Build history of the part. All positions in model axes, mm. A direction names the side the tool comes from. Give positions to 0.01 mm unless a question says otherwise; leave off trailing zeros. Order: outer loops, then holes, each group sorted by start corner. A loop starts at its lowest first (then second) coordinate and runs counter-clockwise, first axis right, second up. Notation, with made-up numbers: (-21, 77.5) - (-4, 77.5) arc R20 ccw to (-4, 107.5) - close; hole circle Ø2 at (42.25, 31.25). An arc over 180 degrees is marked (long way). Use a Markdown table: item, result.
Autodesk Fusion 360 part; units mm, degrees
sketch "Sketch1" plane through (0, 0, 0) normal (0, 0, 1) x (1, 0, 0)
  line L0 (55.4833, 22.0753) -> (95.4833, 22.0753)
  line L1 (95.4833, 22.0753) -> (95.4833, 19.0753)
  line L2 (95.4833, 19.0753) -> (55.4833, 19.0753)
  line L3 (55.4833, 19.0753) -> (55.4833, 22.0753)
  line L4 (95.4833, 22.0753) -> (98.8643, 14.8248)
  line L5 (98.8643, 14.8248) -> (97.7152, 14.289)
  line L6 (97.7152, 14.289) -> (95.4833, 19.0753)
  line L7 (55.4833, 19.0753) -> (50.4119, 29.951)
  line L8 (50.4119, 29.951) -> (51.561, 30.4868)
  line L9 (55.4833, 22.0753) -> (51.561, 30.4868)
  dimension "d2" = 3
  dimension "d3" = 40
  dimension "d5" = 115
  dimension "d8" = 115
  dimension "d9" = 115
  dimension "d10" = 115
  dimension "d12" = 8
  dimension "d13" = 12
extrude "Extrude1" add sketch "Sketch1" along normal blind 12
sketch "Sketch2" plane through (86.8847, 40.515, 0) normal (0.9063, 0.4226, 0) x (-0.4226, 0.9063, 0)
  line L0 (-28.346, 0) -> (-20.346, 0)
  line L1 (-20.346, 0) -> (-20.346, 12)
  line L2 (-20.346, 12) -> (-28.346, 12)
  line L3 (-28.346, 12) -> (-28.346, 0)
  line L4 (-25.346, 12) -> (-25.346, 0) construction
  line L5 (-20.346, 6) -> (-28.346, 6) construction
  circle A0 centre (-25.346, 6) radius 1.1
  dimension "d17" = 2.2
  dimension "d23" = 3
extrude "Extrude2" cut sketch "Sketch2" against normal up to surface (1.2679 mm away) contours A0
sketch "Sketch4" plane through (54.029, 25.1941, 0) normal (0.9063, 0.4226, 0) x (-0.4226, 0.9063, 0)
  line L0 (-3.4413, 0) -> (5.8398, 0)
  line L1 (5.8398, 0) -> (5.8398, 12)
  line L2 (5.8398, 12) -> (-3.4413, 12)
  line L3 (-3.4413, 12) -> (-3.4413, 0)
  line L4 (1.1993, 12) -> (1.1993, 0) construction
  line L5 (5.8398, 6) -> (-3.4413, 6) construction
  circle A0 centre (1.1993, 6) radius 1
  dimension "d24" = 2
extrude "Extrude3" cut sketch "Sketch4" against normal up to surface (1.2679 mm away) contours A0
equation "thickness = 3 mm"
equation "d2 = thickness"
equation "d3 = height"
equation "height = 40 mm"
1) Wall check: line 1 (Y direction, x = 81, z = 2.5); line 2 (X direction, y = 24.25, z = 6); line 3 (Y direction, x = 54, z = 8). Give the ranges that are in metal, low to high. Write a range as from..to.
Computed:
| item | result |
|---|---|
| line 1 | y = 19.08..22.08 |
| line 2 | x = 53.07..54.47 |
| line 3 | y = 22.26..25.26 |
2) Tool access for faces 1 (the flat face through (76, 19.075, 6)), 2 (the flat face through (75, 22.075, 6)), 3 (the flat face through (75, 21, 12)): list every direction of +Z, -Z, +X, -X, +Y, -Y with a clear straight run to the whole face (end or side of a thin tool).
Computed:
| item | result |
|---|---|
| face 1 | +Z, -Z, -X, -Y |
| face 2 | +Z, -Z, +X, +Y |
| face 3 | +Z, +X, -X, +Y, -Y |
3) Pin check, flat tips, straight feed: P1, Ø3.5, axis at x = 85, z = 3.5, coming from the +Y side; P2, Ø2, axis at y = 28.5, z = 8.5, coming from the +X side; P3, Ø1.5, axis at y = 21, z = 8.5, coming from the +X side. Stop position of each tip, or through.
Computed:
| item | result |
|---|---|
| P1 | stops at y = 22.08 |
| P2 | stops at x = 52.95 |
| P3 | stops at x = 96.33 |
4) Slice it at A-A (z = 4). Write the cut outline in (x, y), and give its area (3 significant figures).
Computed:
| item | result |
|---|---|
| outline | (50.41, 29.95) - (55.48, 19.08) - (95.48, 19.08) - (97.72, 14.29) - (98.86, 14.82) - (95.48, 22.08) - (55.48, 22.08) - (51.56, 30.49) - close |
| area | 142 mm² |
5) Slice it at C-C (y = 23.25). Write the cut outline in (x, z).
Computed:
| item | result |
|---|---|
| outline | (53.54, 0) - (54.94, 0) - (54.94, 12) - (53.54, 12) - close |
6) Two-plate mould, pull along Z, no slides. Class faces 4 (the cylindrical face through (97.37, 16.54, 6.74)), 5 (the flat face through (75, 21, 0)), 6 (the flat face through (53, 24.4, 5.9)), 7 (the cylindrical face through (52.55, 26.88, 6.3)): +Z half, -Z half, draft (parallel to the pull), parting line (faces both ways), or undercut.
Computed:
| item | result |
|---|---|
| face 4 | undercut |
| face 5 | -Z half |
| face 6 | draft |
| face 7 | undercut |
7) Slice it at B-B (x = 83). Write the cut outline in (y, z), and give its area (3 significant figures).
Computed:
| item | result |
|---|---|
| outline | (19.08, 0) - (22.08, 0) - (22.08, 12) - (19.08, 12) - close |
| area | 36.0 mm² |
